Autodesk Inventor part; units mm, degrees
ref_plane "Work Plane1" through (33.575, 0, 0) normal (0, 0, -1) x (1, 0, 0)
ref_plane "YZ Plane" through (0, 0, 0) normal (1, 0, 0) x (0, 1, 0)
ref_plane "XZ Plane" through (0, 0, 0) normal (0, 1, 0) x (-1, 0, 0)
sketch "Sketch1" plane through (0, 0, 0) normal (0, 0, 1) x (1, 0, 0)
  line L0 (0, 0) -> (12, 0)
  line L1 (12, 0) -> (12, 1.5)
  line L2 (12, 1.5) -> (2.65, 1.5)
  line L3 (2.65, 1.5) -> (2.3433, 1.1933)
  line L4 (2.3433, 1.1933) -> (1.9567, 1.1933)
  line L5 (1.9567, 1.1933) -> (0.4, 2.75)
  line L6 (0.4, 2.75) -> (0, 2.75)
  line L7 (0, 2.75) -> (0, 0)
  line L8 (2.65, 1.5) -> (1.65, 1.5) construction
  line L9 (-2.4, 0) -> (14.4, 0)
  line L10 (0, 3.3) -> (0, -0.55)
  dimension "d0" = 12
  dimension "d1" = 45
  dimension "d2" = 0.3067
  dimension "d3" = 9.35
  dimension "d4" = 1.65
  dimension "d5" = 2.3866
  dimension "d6" = 3
  dimension "d7" = 5.5
revolve "Body" add sketch "Sketch1" angle 360 about axis through (0, 0, 0) along (1, 0, 0)
sketch "Sketch2" plane through (0, 0, 0) normal (-1, 0, 0) x (0, 0, 1)
  line L0 (2.75, -0.5) -> (-2.75, -0.5)
  line L1 (-2.75, -0.5) -> (-2.75, 0.5)
  line L2 (-2.75, 0.5) -> (2.75, 0.5)
  line L3 (2.75, 0.5) -> (2.75, -0.5)
  line L4 (0, 0.5) -> (0, -0.5) construction
  line L5 (-2.75, 0) -> (2.75, 0) construction
  line L6 (0, 2.75) -> (0, 0)
  dimension "d15" = 1
  dimension "d16" = 5.5
extrude "Slot" cut sketch "Sketch2" against normal blind 0.85
thread "Thread"
chamfer "Chamfer1" distance 0.3067 distance2 0.1534 1 edges at (12, -1.5, 0) measured on face at (12, 0.1505, 0.4164)
ref_plane "Work Plane1" through (33.575, 0, 0) normal (0, 0, -1) x (1, 0, 0)
equation "\"d0\" = NLG"
equation "\"d1\" = 0.5 * SEWI"
equation "\"d2\" = GAL"
equation "\"d3\" = GEL"
equation "\"d4\" = KOH"
equation "\"d5\" = BDM"
equation "\"d6\" = GD"
equation "\"d7\" = KOD"
equation "\"d15\" = SBR"
equation "\"d16\" = KOD"
equation "\"d8\" = STI"
equation "\"d10\" = GEL"
equation "\"d12\" = -0.5 * SPD + 0.5 * GD"
equation "\"d13\" = 0.5 * GAL"
equation "\"NLG\" = 12"
equation "\"GAL\" = 0.61345 * PTC"
equation "\"GEL\" = 9.35"
equation "\"KOH\" = 1.65"
equation "\"KOD\" = 5.5"
equation "\"SEWI\" = 90deg"
equation "\"BDM\" = NND - 1.2269 * PTC"
equation "\"GD\" = NND"
equation "\"SBR\" = 1"
equation "\"STI\" = 0.85"
equation "\"SPD\" = NND - 1.2269 * PTC"
equation "\"GUL\" = 0.61345 * PTC"
equation "\"PTC\" = 0.5"
equation "\"EPV\" = 3.15"
equation "\"THREADDIA\" = 3"
equation "\"TOA\" = 30deg"
equation "\"NND\" = 3"
equation "\"GD1\" = THREADDIA - 1.2269 * PTC"
properties part number "ISO 2009 - M3 x 12" material "Stainless Steel, 440C"
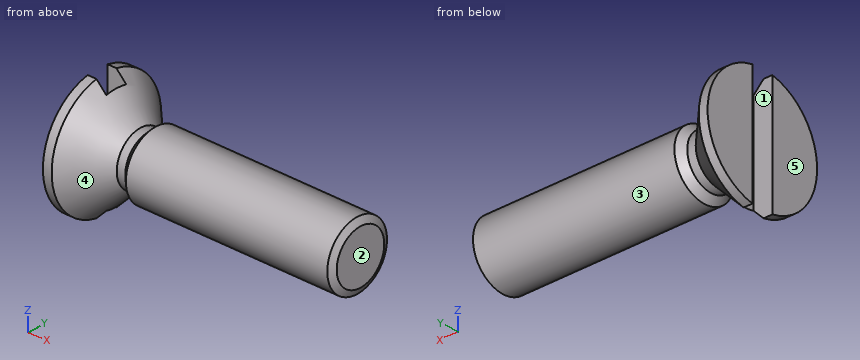
Geometry check sheet. Reference: the model listing, model coordinates, mm. Face numbers are marked on the shaded views. A direction names the side the tool comes from. Give positions to 0.01 mm unless a question says otherwise; leave off trailing zeros. Write each loop counter-clockwise with the first axis right and the second up, starting at its lowest first coordinate (ties: lowest second). Pieces come first, ordered by that corner, then holes.
1) Material ranges on L1, parallel to X at y = -1.3, z = -0.35; L2, parallel to Y at x = 1, z = -0.9; L3, parallel to X at y = -1.95, z = -0.3, recorded low to high.
2) Section check C-C, the plane x = 3.5. Record the boundary of the cut face in (y, z), and give its area (3 significant figures).
3) Release check for a two-part mould opening along Y. For the marked faces 1, 2 and 3 record: pulls with the +Y half, pulls with the -Y half, needs draft (parallel to the pull), parting line crosses it, or undercut.
4) Section check A-A, the plane y = 0. Record the boundary of the cut face in (x, z).
5) Access from +Z, -Z, +X, -X, +Y, -Y to the whole of each face (thin tool, end or side, straight path). Record for the marked faces 4 and 5.
6) Section check B-B, the plane z = 0. Record the boundary of the cut face in (x, y), and give its area (3 significant figures).
7) Gauge pin test, flat ends, axial feed: pin 1 (0.9 mm diameter, centred on x = 0.5, z = 0, fed in from -Y); pin 2 (2 mm diameter, centred on x = 3, z = 0, fed in from -Y); pin 3 (1.5 mm diameter, centred on x = 4.5, y = -1, fed in from -Z); pin 4 (0.8 mm diameter, centred on y = 0, z = -0.5, fed in from -X). Record the tip position at first contact, or that the pin passes through.
Computed:
1. L1: x = 0 to 1.8, 2.5 to 11.92
1. L2: y = -1.95 to 1.95
1. L3: x = 0 to 1.18
2. outline: circle Ø3 at (0, 0)
2. area: 7.07 mm2
3. face 1: undercut
3. face 2: needs draft
3. face 3: parting line crosses it
4. outline: (0.85, -2.3) - (1.96, -1.19) - (2.34, -1.19) - (2.65, -1.5) - (11.85, -1.5) - (12, -1.19) - (12, 1.19) - (11.85, 1.5) - (2.65, 1.5) - (2.34, 1.19) - (1.96, 1.19) - (0.85, 2.3) - close
5. face 4: none
5. face 5: +Z, -Z, -X, +Y, -Y
6. outline: (0, -2.75) - (0.4, -2.75) - (1.96, -1.19) - (2.34, -1.19) - (2.65, -1.5) - (11.85, -1.5) - (12, -1.19) - (12, 1.19) - (11.85, 1.5) - (2.65, 1.5) - (2.34, 1.19) - (1.96, 1.19) - (0.4, 2.75) - (0, 2.75) - (0, 0.5) - (0.85, 0.5) - (0.85, -0.5) - (0, -0.5) - close
6. area: 37.2 mm2
7. pin 1: stops at y = -2.75
7. pin 2: stops at y = -1.5
7. pin 3: stops at z = -1.48
7. pin 4: stops at x = 0.85
